from build123d import *

# Parameters (mm, degrees)
SKETCH_1_R                    = 200
EXTRUDE_251_DEPTH             = 5
CUT_EXTRUDE_3_REACH           = 284.887
SKETCH_2_R                    = 2.6
PATTERN_CIRCULAR_1_COUNT      = 4
SKETCH_4_W                    = 4
SKETCH_4_H                    = 11.5
CUT_REVOLVE_3_ANGLE           = 9.5
CUT_REVOLVE_3_OTHER_WAY_ANGLE = 0.5
FILLET_2_R                    = 1.5
CUT_EXTRUDE_1690_REACH        = 284.887
FILLET_1_R                    = 1.5


with BuildPart() as part:
    # Sketch 1 → Extrude 251 (new body)
    with BuildSketch(Plane(origin=(0, 0, 0), x_dir=(1, 0, 0), z_dir=(0, 1, 0))):
        with Locations(Location((0, 0, 0), (0, 0, 270))):
            Circle(SKETCH_1_R)
    extrude(amount=EXTRUDE_251_DEPTH)

    # Sketch 2 → Cut-Extrude 3 (cut, up to next)
    with BuildSketch(Plane(origin=(0, 5, 0), x_dir=(1, 0, 0), z_dir=(0, 1, 0)), mode=Mode.PRIVATE) as cut_extrude_3_sk1:
        with Locations(Location((0, -175, 0), (0, 0, 270))):
            Circle(SKETCH_2_R)
    cut_extrude_3_tool1 = extrude(cut_extrude_3_sk1.sketch, amount=-CUT_EXTRUDE_3_REACH, mode=Mode.PRIVATE) & part.part
    # Sketch 2 → Cut-Extrude 3 (cut, up to next)
    with BuildSketch(Plane(origin=(0, 5, 0), x_dir=(1, 0, 0), z_dir=(0, 1, 0)), mode=Mode.PRIVATE) as cut_extrude_3_sk2:
        with Locations(Location((0, -187, 0), (0, 0, 270))):
            Circle(SKETCH_2_R)
    cut_extrude_3_tool2 = extrude(cut_extrude_3_sk2.sketch, amount=-CUT_EXTRUDE_3_REACH, mode=Mode.PRIVATE) & part.part
    cut_extrude_3_1 = cut_extrude_3_tool1.solids().sort_by_distance((0, 5, 175))[0]
    add(cut_extrude_3_1, mode=Mode.SUBTRACT)
    cut_extrude_3_2 = cut_extrude_3_tool2.solids().sort_by_distance((0, 5, 187))[0]
    add(cut_extrude_3_2, mode=Mode.SUBTRACT)
    cut_extrude_3 = cut_extrude_3_1 + cut_extrude_3_2  # Cut-Extrude 3 as one shape, for the pattern or mirror that repeats it

    # Pattern Circular 1: Cut-Extrude 3 ×4 about axis
    pattern_circular_1_axis = Axis((0, 0, 0), (0, 1, 0))
    for i in range(1, PATTERN_CIRCULAR_1_COUNT):
        add(cut_extrude_3.rotate(pattern_circular_1_axis, i * 360 / PATTERN_CIRCULAR_1_COUNT), mode=Mode.SUBTRACT)

    # Sketch 4 → Cut-Revolve 3 (revolve, cut)
    with BuildSketch(Plane(origin=(0, 0, 0), x_dir=(0.7036657529829018, 0, -0.710531145045033), z_dir=(0.710531145045033, 0, 0.7036657529829018))):
        with Locations((181.5, 5.25)):
            Rectangle(SKETCH_4_W, SKETCH_4_H)
    revolve(axis=Axis((0, -55, 0), (0, 1, 0)), revolution_arc=CUT_REVOLVE_3_ANGLE, mode=Mode.SUBTRACT)

    # Sketch 4 → Cut-Revolve 3 other way (revolve, cut)
    with BuildSketch(Plane(origin=(0, 0, 0), x_dir=(0.7036657529829018, 0, -0.710531145045033), z_dir=(0.710531145045033, 0, 0.7036657529829018))):
        with Locations((181.5, 5.25)):
            Rectangle(SKETCH_4_W, SKETCH_4_H)
    revolve(axis=Axis((0, -55, 0), (0, -1, 0)), revolution_arc=CUT_REVOLVE_3_OTHER_WAY_ANGLE, mode=Mode.SUBTRACT)

    # Fillet 2
    fillet_2_edges = [part.edges().sort_by_distance(p)[0] for p in [
        (105.832512271, 2.5, -149.905734868),
        (103.525536527, 2.5, -146.638034926),
    ]]
    fillet(fillet_2_edges, radius=FILLET_2_R)

    # Sketch 6 → Cut-Extrude 1690 (cut, up to next)
    with BuildSketch(Plane(origin=(0, 5, 0), x_dir=(1, 0, 0), z_dir=(0, 1, 0)), mode=Mode.PRIVATE) as cut_extrude_1690_sk1:
        with BuildLine():
            Line((122.328963701, 123.036070482), (133.642715214, 134.349821995))
            ThreePointArc((133.642715214, 134.349821995), (135.160960115, 132.822305585), (136.66174685, 131.277633083))
            Line((136.66174685, 131.277633083), (125.152266287, 120.163056899))
            ThreePointArc((125.152266287, 120.163056899), (123.748952928, 121.607757356), (122.328963701, 123.036070482))
        make_face()
    cut_extrude_1690_tool1 = extrude(cut_extrude_1690_sk1.sketch, amount=-CUT_EXTRUDE_1690_REACH, mode=Mode.PRIVATE) & part.part
    add(cut_extrude_1690_tool1.solids().sort_by_distance((129.515831, 5, -127.274853))[0], mode=Mode.SUBTRACT)

    # Fillet 1
    fillet_1_edges = [part.edges().sort_by_distance(p)[0] for p in [
        (125.152266287, 2.5, -120.163056899),
        (122.328963701, 2.5, -123.036070482),
        (133.642715214, 2.5, -134.349821995),
        (136.66174685, 2.5, -131.277633083),
    ]]
    fillet(fillet_1_edges, radius=FILLET_1_R)


solid = part.part
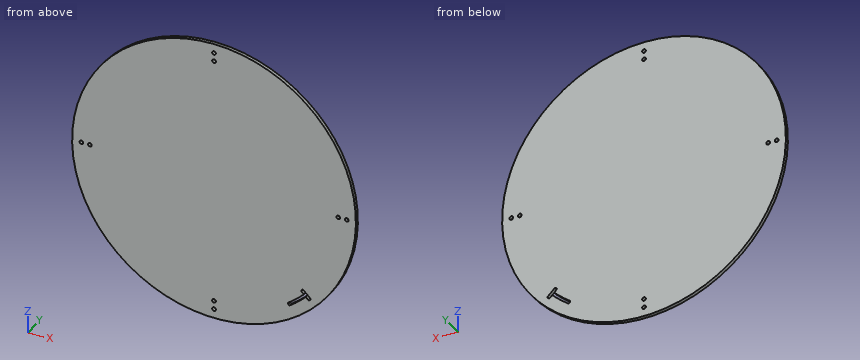
Part model, mm, in its own coordinate system. Coordinates: 2 decimals unless noted, no trailing zeros. Loops run counter-clockwise (first coordinate to the right, second up) from the corner with the lowest first, then second, coordinate; pieces in that order, holes last. Notation, with made-up numbers: M 19.5,-37.5 L 60.5,-37.5 A14 ccw 60.5,-32.5 Z; hole C 78.25,46 d8. An arc over 180 degrees is marked long. Use a Markdown table: item, result. Add a question column.
Q1. Cut at B-B (x = 77). Write the cut outline in (y, z).
Q2. Probe L1, parallel to X at y = 4.35, z = -127; L2, parallel to Z at x = -175, y = 1.55; L3, parallel to X at y = 3.2, z = -47. List the from-to ranges inside material, lowest first.
Q3. Cut at A-A (y = 2.3). Give the number of separate pieces and of enclosed holes in the cut face, and give its area (3 significant figures).
Q4. Pin check, flat tips, straight feed: P1, Ø1, axis at y = 2, z = -93, coming from the +X side; P2, Ø1.5, axis at y = 3.5, z = -105, coming from the -X side; P3, Ø4.5, axis at x = -187, z = 0, coming from the +Y side. Stop position of each tip, or through.
Q5. Cut at C-C (z = -96). Write the cut outline in (x, y).
Worked out:
| question | item | result |
|---|---|---|
| 1 | outline | M 0,-184.58 L 5,-184.58 L 5,184.58 L 0,184.58 Z |
| 2 | L1 | x = -154.5 to 126.29, 132.23 to 154.5 |
| 2 | L2 | z = -96.82 to -2.6, 2.6 to 96.82 |
| 2 | L3 | x = -194.4 to 194.4 |
| 3 | separate pieces | 1 |
| 3 | enclosed holes | 9 |
| 3 | area | 125,000 mm2 |
| 4 | P1 | stops at x = 177.32 |
| 4 | P2 | stops at x = -170.68 |
| 4 | P3 | passes through |
| 5 | outline | M -175.45,0 L 175.45,0 L 175.45,5 L -175.45,5 Z |
